```python
from build123d import *

# Parameters (mm, degrees)
SKETCH1_R           = 41.75125
BOSS_EXTRUDE1_DEPTH = 6.35
SKETCH2_R           = 2.38125
BOSS_EXTRUDE2_DEPTH = 3.175
SKETCH3_R           = 79.85125
BOSS_EXTRUDE3_DEPTH = 6.35
SKETCH4_R           = 2.38125
BOSS_EXTRUDE4_DEPTH = 4.7625
SKETCH5_R           = 77.31125
BOSS_EXTRUDE5_DEPTH = 38.1
FILLET1_R           = 2.54
CUT_EXTRUDE1_DEPTH  = 38.1
SKETCH8_R           = 3.81
CUT_EXTRUDE2_DEPTH  = 97.536
SKETCH9_R           = 6.35
CUT_EXTRUDE3_DEPTH  = 50.8
SKETCH10_R          = 11.1125
CUT_EXTRUDE4_DEPTH  = 19.05
SKETCH11_W          = 6.35
SKETCH11_H          = 12.7
CUT_EXTRUDE5_DEPTH  = 25.4
SKETCH12_R          = 11.1125
SKETCH12_R_2        = 6.35
BOSS_EXTRUDE6_DEPTH = 6.35


with BuildPart() as part:
    # Sketch1 → Boss-Extrude1 (new body)
    with BuildSketch(Plane(origin=(0, 0, 0), x_dir=(1, 0, 0), z_dir=(0, 1, 0))):
        with Locations(Location((0, 0, 0), (0, 0, 270))):
            Circle(SKETCH1_R)
    extrude(amount=BOSS_EXTRUDE1_DEPTH)

    # Sketch2 → Boss-Extrude2 (add)
    with BuildSketch(Plane(origin=(0, 6.35, 0), x_dir=(1, 0, 0), z_dir=(0, 1, 0))):
        with Locations(Location((0, 39.37, 0), (0, 0, 89.99945926))):
            Circle(SKETCH2_R)
        with Locations(Location((27.838793975, 27.838793975, 0), (0, 0, 44.999445214))):
            Circle(SKETCH2_R)
        with Locations(Location((39.37, 0, 0), (0, 0, 359.999429558))):
            Circle(SKETCH2_R)
        with Locations(Location((27.838793975, -27.838793975, 0), (0, 0, 314.999421479))):
            Circle(SKETCH2_R)
        with Locations(Location((0, -39.37, 0), (0, 0, 269.999424945))):
            Circle(SKETCH2_R)
        with Locations(Location((-27.838793975, -27.838793975, 0), (0, 0, 224.999438328))):
            Circle(SKETCH2_R)
        with Locations(Location((-39.37, 0, 0), (0, 0, 179.999453674))):
            Circle(SKETCH2_R)
        with Locations(Location((-27.838793975, 27.838793975, 0), (0, 0, 134.999462078))):
            Circle(SKETCH2_R)
    extrude(amount=BOSS_EXTRUDE2_DEPTH)

    # Sketch3 → Boss-Extrude3 (add)
    with BuildSketch(Plane.XZ):
        with Locations(Location((0, 0, 0), (0, 0, 270))):
            Circle(SKETCH3_R)
    extrude(amount=BOSS_EXTRUDE3_DEPTH)

    # Sketch4 → Boss-Extrude4 (add)
    with BuildSketch(Plane(origin=(0, 0, 0), x_dir=(1, 0, 0), z_dir=(0, 1, 0))):
        with Locations(Location((0, 77.47, 0), (0, 0, 89.999466901))):
            Circle(SKETCH4_R)
        with Locations(Location((67.090988031, 38.735, 0), (0, 0, 29.999456844))):
            Circle(SKETCH4_R)
        with Locations(Location((67.090988031, -38.735, 0), (0, 0, 329.999448342))):
            Circle(SKETCH4_R)
        with Locations(Location((0, -77.47, 0), (0, 0, 270))):
            Circle(SKETCH4_R)
        with Locations(Location((-67.090988031, -38.735, 0), (0, 0, 209.999457825))):
            Circle(SKETCH4_R)
        with Locations(Location((-67.090988031, 38.735, 0), (0, 0, 149.999465475))):
            Circle(SKETCH4_R)
    extrude(amount=BOSS_EXTRUDE4_DEPTH)

    # Sketch5 → Boss-Extrude5 (add)
    with BuildSketch(Plane.XZ.offset(6.35)):
        with Locations(Location((0, 0, 0), (0, 0, 90))):
            Circle(SKETCH5_R)
    extrude(amount=BOSS_EXTRUDE5_DEPTH)

    # Sketch6 → Revolve1 (revolve)
    with BuildSketch(Plane(origin=(0, 0, 0), x_dir=(0, 0, -1), z_dir=(1, 0, 0)), mode=Mode.PRIVATE) as revolve1_sk:
        Polygon((77.31125, -6.35), (77.31125, -44.45), (79.85125, -6.35), align=None)
    revolve(revolve1_sk.sketch.rotate(Axis((0, 12.22375, 0), (0, -1, 0)), 180), axis=Axis((0, 12.22375, 0), (0, -1, 0)))

    # Fillet1
    # the kernel refuses this fillet: 2.54 mm, written as the material it takes off along each edge
    with BuildSketch(Plane(origin=(0, -6.35, 0), x_dir=(0, 0, 1), z_dir=(1, 0, 0))) as fillet1_piece_1:
        with BuildLine():
            CenterArc((79.85125 - FILLET1_R, -FILLET1_R * 0.0332963783729), FILLET1_R, 0, 3.814074834)
            Line((79.85125 - FILLET1_R * 0.00221484214339, FILLET1_R * 0.0332226321509), (79.85125, 0))
            Line((79.85125, 0), (79.85125, -FILLET1_R * 0.0332963783729))
        make_face()
    revolve(axis=Axis((0, -6.35, 0), (0, -1, 0)), revolution_arc=180, mode=Mode.SUBTRACT)
    with BuildSketch(Plane(origin=(0, -6.35, 0), x_dir=(0, 0, -1), z_dir=(-1, 0, 0))) as fillet1_piece_2:
        with BuildLine():
            CenterArc((79.85125 - FILLET1_R, -FILLET1_R * 0.0332963783729), FILLET1_R, 0, 3.814074834)
            Line((79.85125 - FILLET1_R * 0.00221484214339, FILLET1_R * 0.0332226321509), (79.85125, 0))
            Line((79.85125, 0), (79.85125, -FILLET1_R * 0.0332963783729))
        make_face()
    revolve(axis=Axis((0, -6.35, 0), (0, -1, 0)), revolution_arc=180, mode=Mode.SUBTRACT)

    # Sketch7 → Cut-Extrude1 (cut)
    with BuildSketch(Plane.XZ.offset(44.45)):
        Polygon((48.768, -31.75), (48.768, 31.75), (70.490899246, 31.75), (86.685802419, 31.75), (86.685802419, -31.75), (70.490899246, -31.75), align=None)
        Polygon((-48.768, -31.75), (-48.768, 31.75), (-70.490899246, 31.75), (-86.531926913, 31.75), (-86.531926913, -31.75), (-70.490899246, -31.75), align=None)
    extrude(amount=-CUT_EXTRUDE1_DEPTH, mode=Mode.SUBTRACT)

    # Sketch8 → Cut-Extrude2 (cut)
    with BuildSketch(Plane.ZY.offset(48.768)):
        with Locations((0, -25.4)):
            Circle(SKETCH8_R)
    extrude(amount=-CUT_EXTRUDE2_DEPTH, mode=Mode.SUBTRACT)

    # Sketch9 → Cut-Extrude3 (cut)
    with BuildSketch(Plane(origin=(0, 6.35, 0), x_dir=(1, 0, 0), z_dir=(0, 1, 0))):
        with Locations(Location((0, 0, 0), (0, 0, 270))):
            Circle(SKETCH9_R)
    extrude(amount=-CUT_EXTRUDE3_DEPTH, mode=Mode.SUBTRACT)

    # Sketch10 → Cut-Extrude4 (cut)
    with BuildSketch(Plane.XZ.offset(44.45)):
        with Locations(Location((0, 0, 0), (0, 0, 270))):
            Circle(SKETCH10_R)
    extrude(amount=-CUT_EXTRUDE4_DEPTH, mode=Mode.SUBTRACT)

    # Sketch11 → Cut-Extrude5 (cut)
    with BuildSketch(Plane.XZ.offset(44.45)):
        with Locations((36.968003166, 0.307880226)):
            Rectangle(SKETCH11_W, SKETCH11_H)
        with Locations((-36.968003166, 0.307880226)):
            Rectangle(SKETCH11_W, SKETCH11_H)
    extrude(amount=-CUT_EXTRUDE5_DEPTH, mode=Mode.SUBTRACT)

    # Sketch12 → Boss-Extrude6 (add)
    with BuildSketch(Plane.XZ.offset(25.4)):
        with Locations(Location((0, 0, 0), (0, 0, 270))):
            Circle(SKETCH12_R)
        with Locations(Location((0, 0, 0), (0, 0, 90))):
            Circle(SKETCH12_R_2, mode=Mode.SUBTRACT)
    extrude(amount=-BOSS_EXTRUDE6_DEPTH)


solid = part.part
```
The model under review builds one solid part; all positions refer to its coordinate system, in mm. A direction names the side the tool comes from. Give positions to 0.01 mm unless a question says otherwise; leave off trailing zeros. Write each loop counter-clockwise with the first axis right and the second up, starting at its lowest first coordinate (ties: lowest second). Pieces come first, ordered by that corner, then holes. Notation, with made-up numbers: (86, 20.5) - (136, 20.5) arc R21 cw to (136, 26.5) - close; hole circle Ø7 at (55.25, 9). An arc over 180 degrees is marked (long way). Answer in a Markdown table with one row per item. Add a question column.
1. We need section A-A on y = -36. State how many separate pieces and enclosed holes the cut face has, then the cut area to 3 significant figures.
2. Draft analysis for pull direction Z (two halves, no side actions). For faces 4 (the cylindrical face through (0.1, 7.92, 36.99)), 5 (the flat face through (-28, 9.525, -28)), 6 (the cylindrical face through (-11.112, -23.94, 0.054)), state which applies: +Z half, -Z half, draft (parallel to the pull), parting line (faces both ways), or undercut.
3. Tool access review of faces 1 (the cylindrical face through (0.1, 2.35, 75.09)), 2 (the flat face through (-67, 4.762, 39)), 3 (the flat face through (37, -32, 6.658)): name each direction out of +Z, -Z, +X, -X, +Y, -Y from which nothing blocks a thin tool from reaching the whole face with its end or side.
4. Wall thickness on line 1 along Y through (x, z) = (-42.5, 0); line 2 along X through (y, z) = (-31, 0); line 3 along Y through (x, z) = (26, 0): over which ranges is each line inside the solid? List them lowest first. Write a range as [from, to].
5. We need section B-B on y = -13.5. Write out the cut boundary in (x, z).
6. Insertion check: P1, Ø2, axis at y = -6, z = -58.5, coming from the +X side; P2, Ø6.5, axis at y = -26.5, z = -0.5, coming from the -X side; P3, Ø2.5, axis at x = -66.5, z = 38.5, coming from the +Y side; P4, Ø3, axis at x = -25.5, z = -25, coming from the +Y side (3 decimals). Each pin has a flat end and moves straight along its axis. Give the tip position at first contact, or say it passes through.
Ans:
| question | item | result |
|---|---|---|
| 1 | separate pieces | 1 |
| 1 | enclosed holes | 3 |
| 1 | area | 15,100 mm^2 |
| 2 | face 4 | undercut |
| 2 | face 5 | draft |
| 2 | face 6 | undercut |
| 3 | face 1 | +Y |
| 3 | face 2 | +Z, -Z, -X, +Y |
| 3 | face 3 | -Y |
| 4 | line 1 | y = [-44.45, -29.21], [-21.59, 0] |
| 4 | line 2 | x = [-48.77, -40.14], [-33.79, -11.11], [11.11, 33.79], [40.14, 48.77] |
| 4 | line 3 | y = [-44.45, -29.21], [-21.59, 6.35] |
| 5 | outline | (-72.75, -31.75) arc R79.37 ccw to (72.75, -31.75) - (48.77, -31.75) - (48.77, 31.75) - (72.75, 31.75) arc R79.37 ccw to (-72.75, 31.75) - (-48.77, 31.75) - (-48.77, -31.75) - close; hole circle Ø12.7 at (0, 0) |
| 6 | P1 | stops at x = 55.41 |
| 6 | P2 | stops at x = -48.77 |
| 6 | P3 | stops at y = 4.76 |
| 6 | P4 | stops at y = 9.525 |
